CAD build for the part. Positions are in the model's coordinates, mm. Coordinates: 2 decimals unless noted, no trailing zeros. Order: outer loops, then holes, each group sorted by start corner. A loop starts at its lowest first (then second) coordinate and runs counter-clockwise, first axis right, second up. Notation, with made-up numbers: (20.25, 16) - (34.25, 16) arc R14 ccw to (34.25, 37) - close; hole circle Ø2 at (51, -26.5). An arc over 180 degrees is marked (long way). Use one line per item in the form item = value.
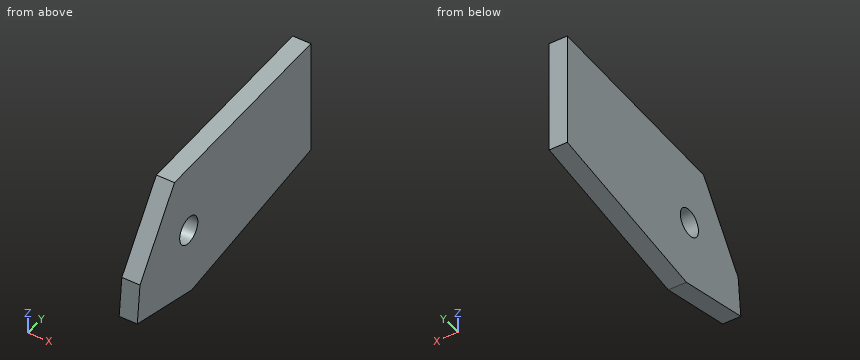
Autodesk Inventor part; units mm, degrees
ref_plane "YZ Plane" through (0, 0, 0) normal (1, 0, 0) x (0, 1, 0)
ref_plane "XZ Plane" through (0, 0, 0) normal (0, 1, 0) x (-1, 0, 0)
ref_plane "XY Plane" through (0, 0, 0) normal (0, 0, 1) x (1, 0, 0)
sketch "Sketch1" plane through (0, 0, 0) normal (1, 0, 0) x (0, 1, 0)
  line L0 (0, 0) -> (0, -32.004)
  line L1 (6.1409, 0) -> (6.1409, -25.4) construction
  line L2 (0, -32.004) -> (-50.0461, -40.0442)
  line L3 (-50.0461, -40.0442) -> (-72.9333, -34.7254)
  line L4 (-72.9333, -34.7254) -> (-71.805, -23.7653)
  line L5 (-71.805, -23.7653) -> (-57.2991, -2.8123)
  line L6 (-57.2991, -2.8123) -> (0, 0)
  circle A0 centre (-51.308, -21.2399) radius 3.81
  dimension "d0" = 32.004
  dimension "d1" = 25.4
  dimension "d2" = 7.62
  dimension "d3" = 51.308
extrude "Extrusion1" add sketch "Sketch1" along normal blind 5.08
properties part number "Handle Insert V1"
Item 1: Drop a flat-ended pin along its axis: pin 1 (1.5 mm diameter, centred on x = 1.5, y = -57, fed in from +Z). Give the stop position or say it passes through.
Derived:
pin_1 = -2.76
Item 2: Cut at C-C, the plane y = -38. Write the cut outline in (x, z), plus the area to 3 significant figures.
Derived:
outline = (0, -38.11) - (5.08, -38.11) - (5.08, -1.87) - (0, -1.87) - close
area = 184 mm²
Item 3: Cut at A-A, the plane z = -22. Write the cut outline in (x, y), plus the area to 3 significant figures.
Derived:
outline = (0, -70.58) - (5.08, -70.58) - (5.08, -55.04) - (0, -55.04) - close; (0, -47.57) - (5.08, -47.57) - (5.08, 0) - (0, 0) - close
area = 321 mm²
Item 4: Cut at D-D, the plane z = -33.5. Write the cut outline in (x, y).
Derived:
outline = (0, -72.81) - (5.08, -72.81) - (5.08, -9.31) - (0, -9.31) - close
Item 5: Drill centre lines: line 1 (Y direction, x = 3.75, z = -20.5); line 2 (Z direction, x = 2.5, y = -14); line 3 (Z direction, x = 4.75, y = -6.5). Where is each one in solid material? Low to high. Write a range as [from, to].
Derived:
line_1 = [-69.54, -55.05], [-47.57, 0]
line_2 = [-34.25, -0.69]
line_3 = [-33.05, -0.32]
Item 6: Cut at B-B, the plane x = 1.45. Write the cut outline in (y, z) (3 decimals), plus the area to 3 significant figures.
Derived:
outline = (-72.933, -34.725) - (-50.046, -40.044) - (0, -32.004) - (0, 0) - (-57.299, -2.812) - (-71.805, -23.765) - close; hole circle Ø7.62 at (-51.308, -21.24)
area = 2,310 mm²
